```python
from build123d import *

# Parameters (mm, degrees)
SKETCH1_R           = 4.05
BOSS_EXTRUDE1_DEPTH = 10
SKETCH3_W           = 50
SKETCH3_H           = 50
CUT_EXTRUDE2_DEPTH  = 15
SKETCH4_W           = 40
SKETCH4_H           = 40
CUT_EXTRUDE3_DEPTH  = 132.363046554
FILLET1_R           = 2.5


with BuildPart() as part:
    # Sketch1 → Boss-Extrude1 (new, symmetric)
    with BuildSketch(Plane.XY):
        with BuildLine():
            Line((-77.5, 0), (77.5, 0))
            Line((77.5, 0), (77.5, 7.5))
            ThreePointArc((77.5, 7.5), (75.303300859, 12.803300859), (70, 15))
            Line((70, 15), (25, 15))
            Line((25, 15), (25, 105))
            Line((25, 105), (-25, 105))
            Line((-25, 105), (-25, 15))
            Line((-25, 15), (-70, 15))
            ThreePointArc((-70, 15), (-75.303300859, 12.803300859), (-77.5, 7.5))
            Line((-77.5, 7.5), (-77.5, 0))
        make_face()
        with Locations((-70, 7.5)):
            Circle(SKETCH1_R, mode=Mode.SUBTRACT)
        with Locations((70, 7.5)):
            Circle(SKETCH1_R, mode=Mode.SUBTRACT)
    extrude(amount=BOSS_EXTRUDE1_DEPTH, both=True)

    # Sketch3 → Cut-Extrude2 (cut)
    with BuildSketch(Plane.XY.offset(10)):
        with Locations((0, 80)):
            Rectangle(SKETCH3_W, SKETCH3_H)
    extrude(amount=-CUT_EXTRUDE2_DEPTH, mode=Mode.SUBTRACT)

    # Sketch4 → Cut-Extrude3 (cut, through all)
    with BuildSketch(Plane.XY.offset(-5)):
        with Locations((0, 80)):
            Rectangle(SKETCH4_W, SKETCH4_H)
    extrude(amount=-CUT_EXTRUDE3_DEPTH, mode=Mode.SUBTRACT)

    # Fillet1
    fillet1_edges = [part.edges().sort_by_distance(p)[0] for p in [
        (-20, 60, -7.5),
        (-20, 100, -7.5),
        (20, 100, -7.5),
        (20, 60, -7.5),
    ]]
    fillet(fillet1_edges, radius=FILLET1_R)


solid = part.part
```
Design review of the part built by this model. Coordinates are the model's own, in mm. A direction names the side the tool comes from. Give positions to 0.01 mm unless a question says otherwise; leave off trailing zeros. Order: outer loops, then holes, each group sorted by start corner. A loop starts at its lowest first (then second) coordinate and runs counter-clockwise, first axis right, second up. Notation, with made-up numbers: (68.25, -34) -> (73.25, -34) arc R18 cw to (73.25, -3) -> close; hole circle Ø8 at (-11.5, 64). An arc over 180 degrees is marked (long way). Write each question's results on one line, items separated by ' | '. Start each with the question number.
Q1. Add section C-C on z = 7.25. Give the boundary of the cut face in (x, y), and give its area (3 significant figures).
Q2. Add section B-B on y = 94. Give the boundary of the cut face in (x, z), and give its area (3 significant figures).
Q3. Add section D-D on z = -8. Give the boundary of the cut face in (x, y).
Q4. Machinability: for faces 1 (the flat face through (-47, 15, 0)), 2 (the flat face through (-77.5, 4, 0)), 3 (the flat face through (0, 103, -5)), 4 (the flat face through (25, 39, -2)), 5 (the flat face through (-20, 80, -7)), which of the approach directions +Z, -Z, +X, -X, +Y, -Y give a long, thin tool a straight path to every point of the face, cutting with its end or side? Answer none if there is none.
Q5. Add section A-A on x = 5. Give the boundary of the cut face in (y, z).
Q6. For pin 1 (12 mm diameter, centred on x = 11.5, z = 2.5, fed in from +Y); pin 2 (4 mm diameter, centred on y = 54, z = -3.5, fed in from -X); pin 3 (1.5 mm diameter, centred on y = 87.5, z = -8, fed in from +X), all flat-tipped, find the tip position at first contact; note any pin that passes through.
Q7. Wall thickness on L1, parallel to X at y = 90, z = -8.75; L2, parallel to Y at x = 15, z = -8.5; L3, parallel to X at y = 6.5, z = -7.5: over which ranges is each line inside the solid? List them lowest first. Write a range as from..to.
Q8. Mouldability with a two-part tool opening along Y and no side actions: class faces 6 (the flat face through (-1, 22, 10)), 7 (the flat face through (0, 105, -7)), 8 (the flat face through (20, 80, -7)) as +Y half, -Y half, draft (parallel to the pull), parting line (faces both ways), or undercut.
Found:
1) outline: (-77.5, 0) -> (77.5, 0) -> (77.5, 7.5) arc R7.5 ccw to (70, 15) -> (25, 15) -> (25, 55) -> (-25, 55) -> (-25, 15) -> (-70, 15) arc R7.5 ccw to (-77.5, 7.5) -> close; hole circle Ø8.1 at (-70, 7.5); hole circle Ø8.1 at (70, 7.5) | area: 4,200 mm2
2) outline: (-25, -10) -> (-20, -10) -> (-20, -5) -> (-25, -5) -> close; (20, -10) -> (25, -10) -> (25, -5) -> (20, -5) -> close | area: 50.0 mm2
3) outline: (-77.5, 0) -> (77.5, 0) -> (77.5, 7.5) arc R7.5 ccw to (70, 15) -> (25, 15) -> (25, 105) -> (-25, 105) -> (-25, 15) -> (-70, 15) arc R7.5 ccw to (-77.5, 7.5) -> close; hole circle Ø8.1 at (-70, 7.5); hole (-20, 62.5) arc R2.5 ccw to (-17.5, 60) -> (17.5, 60) arc R2.5 ccw to (20, 62.5) -> (20, 97.5) arc R2.5 ccw to (17.5, 100) -> (-17.5, 100) arc R2.5 ccw to (-20, 97.5) -> close; hole circle Ø8.1 at (70, 7.5)
4) face 1: +Z, -Z, -X, +Y | face 2: +Z, -Z, -X, +Y, -Y | face 3: +Z, +X, -X, +Y | face 4: +Z, -Z, +X, +Y | face 5: +Z, -Z
5) outline: (0, -10) -> (60, -10) -> (60, -5) -> (55, -5) -> (55, 10) -> (0, 10) -> close; (100, -10) -> (105, -10) -> (105, -5) -> (100, -5) -> close
6) pin 1: stops at y = 55 | pin 2: stops at x = -25 | pin 3: stops at x = 25
7) L1: x = -25..-20, 20..25 | L2: y = 0..60, 100..105 | L3: x = -77.5..-73.92, -66.08..66.08, 73.92..77.5
8) face 6: draft | face 7: +Y half | face 8: undercut
